```python
from build123d import *

# Parameters (mm, degrees)
BOSS_EXTRUDE1_DEPTH  = 7.1
SKETCH2_R            = 0.714611453
SKETCH2_R_2          = 0.75
BOSS_EXTRUDE2_DEPTH  = 0.48
SKETCH8_R            = 0.75
BOSS_EXTRUDE4_DEPTH  = 0.48
SKETCH9_R            = 0.75
BOSS_EXTRUDE5_DEPTH  = 0.48
SKETCH10_R           = 0.714611453
SKETCH10_R_2         = 0.75
BOSS_EXTRUDE7_DEPTH  = 0.48
SKETCH11_R           = 0.714611453
SKETCH11_R_2         = 0.75
BOSS_EXTRUDE8_DEPTH  = 0.48
SKETCH12_R           = 0.714611453
BOSS_EXTRUDE9_DEPTH  = 0.48
SKETCH13_R           = 0.75
BOSS_EXTRUDE10_DEPTH = 0.48
SKETCH15_R           = 1.5875
CUT_EXTRUDE3_DEPTH   = 8.1


with BuildPart() as part:
    # Sketch1 → Boss-Extrude1 (new body)
    with BuildSketch(Plane.XY):
        Polygon((-0.007801135, 4.977998784), (-3.525492932, 3.514460461), (-4.977998784, -0.007801135), (-3.514460461, -3.525492932), (0.007801135, -4.977998784), (3.525492932, -3.514460461), (4.977998784, 0.007801135), (3.514460461, 3.525492932), align=None)
    extrude(amount=BOSS_EXTRUDE1_DEPTH)

    # Sketch2 → Boss-Extrude2 (add)
    with BuildSketch(Plane(origin=(1.753329663, 4.251745858, 0), x_dir=(0.924478109, -0.381235132, 0), z_dir=(0.381235132, 0.924478109, 0))):
        with Locations((0, -1.25)):
            Circle(SKETCH2_R)
        with Locations((0, -3.55)):
            Circle(SKETCH2_R_2)
        with Locations((0, -5.85)):
            Circle(SKETCH2_R_2)
    extrude(amount=BOSS_EXTRUDE2_DEPTH)

    # Sketch8 → Boss-Extrude4 (add)
    with BuildSketch(Plane(origin=(4.246229622, 1.766647033, 0), x_dir=(0, 0, -1), z_dir=(0.923278687, 0.384130793, 0))):
        with Locations((-3.55, 0)):
            Circle(SKETCH8_R)
        with Locations((-5.85, 0)):
            Circle(SKETCH8_R)
    extrude(amount=BOSS_EXTRUDE4_DEPTH)

    # Sketch9 → Boss-Extrude5 (add)
    with BuildSketch(Plane(origin=(4.251745858, -1.753329663, 0), x_dir=(0, 0, -1), z_dir=(0.924478109, -0.381235132, 0))):
        with Locations((-5.85, 0)):
            Circle(SKETCH9_R)
    extrude(amount=BOSS_EXTRUDE5_DEPTH)

    # Sketch10 → Boss-Extrude7 (add)
    with BuildSketch(Plane(origin=(1.766647033, -4.246229622, 0), x_dir=(0.923278687, 0.384130793, 0), z_dir=(0.384130793, -0.923278687, 0))):
        with Locations((0, 5.85)):
            Circle(SKETCH10_R)
        with Locations((0, 1.25)):
            Circle(SKETCH10_R_2)
    extrude(amount=BOSS_EXTRUDE7_DEPTH)

    # Sketch11 → Boss-Extrude8 (add)
    with BuildSketch(Plane(origin=(-1.766647033, 4.246229622, 0), x_dir=(0.923278687, 0.384130793, 0), z_dir=(-0.384130793, 0.923278687, 0))):
        with Locations((-0.048036035, -1.25)):
            Circle(SKETCH11_R)
        with Locations((-0.048036035, -3.55)):
            Circle(SKETCH11_R_2)
    extrude(amount=BOSS_EXTRUDE8_DEPTH)

    # Sketch12 → Boss-Extrude9 (add)
    with BuildSketch(Plane(origin=(-4.251745858, 1.753329663, 0), x_dir=(0, 0, 1), z_dir=(-0.924478109, 0.381235132, 0))):
        with Locations((1.25, 0)):
            Circle(SKETCH12_R)
    extrude(amount=BOSS_EXTRUDE9_DEPTH)

    # Sketch13 → Boss-Extrude10 (add)
    with BuildSketch(Plane(origin=(-1.753329663, -4.251745858, 0), x_dir=(0.924478109, -0.381235132, 0), z_dir=(-0.381235132, -0.924478109, 0))):
        with Locations((0, 3.55)):
            Circle(SKETCH13_R)
    extrude(amount=BOSS_EXTRUDE10_DEPTH)

    # Sketch15 → Cut-Extrude3 (cut, through all)
    with BuildSketch(Plane.XY.offset(7.1)):
        Circle(SKETCH15_R)
    extrude(amount=-CUT_EXTRUDE3_DEPTH, mode=Mode.SUBTRACT)


solid = part.part
```
Geometry check sheet. Reference: the model listing, model coordinates, mm. Round coordinates to 2 decimals unless told otherwise and drop trailing zeros. Loops run counter-clockwise (first coordinate to the right, second up) from the corner with the lowest first, then second, coordinate; pieces in that order, holes last. Notation, with made-up numbers: (46, -33.75) - (95, -33.75) arc R19 ccw to (95, -23.75) - close; hole circle Ø4 at (54, 24.5). An arc over 180 degrees is marked (long way). Write item = value, one per line. Start each with the question number.
1. Section check A-A on x = -0.25. Enter the section's corners in (y, z).
2. Section check C-C on y = 3.75. Enter the section's corners in (x, z).
3. Section check B-B on z = 6. Enter the section's corners in (x, y) (1 decimal), then the cut area to 3 significant figures.
4. Section check D-D on z = 0.75. Enter the section's corners in (x, y) (1 decimal).
5. Thickness scan on line 1 (Y direction, x = 0, z = 3.5); line 2 (Y direction, x = 0.75, z = 1.5); line 3 (X direction, y = 0.5, z = 4.75). Record the ranges inside material, lowest first.
6. Depth check by flat-ended pin: pin 1 (3 mm diameter, centred on x = -2.5, z = 4.5, fed in from +Y); pin 2 (1.5 mm diameter, centred on y = 1, z = 3.5, fed in from -X); pin 3 (3 mm diameter, centred on y = -0.5, z = 6, fed in from +X). Enter the tip coordinate at first touch or a pass-through.
7. Mould release check, pull along Z, two halves, no side actions. Record for faces 1 (the face through (1.941, -4.693, 1.26)), 2 (the face through (-1.182, -4.743, 3.775)), 3 (the face through (1.742, -4.256, 3.5)): released by +Z, released by -Z, zero draft, split by the parting line, or undercut.
Working result:
q1.outline = (-4.87, 0) - (-1.57, 0) - (-1.57, 7.1) - (-4.87, 7.1) - close; (1.57, 0) - (4.88, 0) - (4.88, 7.1) - (1.57, 7.1) - close
q2.outline = (-2.96, 0) - (2.97, 0) - (2.97, 7.1) - (-2.96, 7.1) - close
q3.outline = (-5, 0) - (-3.5, -3.5) - (0, -5) - (1.1, -4.5) - (1.3, -5) - (2.6, -4.4) - (2.4, -4) - (3.5, -3.5) - (4, -2.4) - (4.4, -2.6) - (5, -1.3) - (4.5, -1.1) - (5, 0) - (4.5, 1.1) - (5, 1.3) - (4.4, 2.6) - (4, 2.4) - (3.5, 3.5) - (2.4, 4) - (2.6, 4.4) - (1.3, 5) - (1.1, 4.5) - (0, 5) - (-3.5, 3.5) - close; hole circle Ø3.2 at (0, 0)
q3.area = 65.0 mm^2
q4.outline = (-5, 0) - (-3.5, -3.5) - (0, -5) - (1.3, -4.5) - (1.4, -4.9) - (2.5, -4.5) - (2.3, -4) - (3.5, -3.5) - (5, 0) - (3.5, 3.5) - (2.2, 4.1) - (2.4, 4.5) - (1.5, 4.9) - (1.3, 4.4) - (0, 5) - (-1.3, 4.4) - (-1.5, 4.9) - (-2.5, 4.5) - (-2.3, 4) - (-3.5, 3.5) - (-4.1, 2.2) - (-4.5, 2.4) - (-4.9, 1.5) - (-4.4, 1.3) - close; hole circle Ø3.2 at (0, 0)
q5.line_1 = -4.97 to -1.59, 1.59 to 4.97
q5.line_2 = -4.67 to -1.4, 1.4 to 4.67
q5.line_3 = -4.77 to -1.51, 1.51 to 4.77
q6.pin_1 = 4.96
q6.pin_2 = -4.87
q6.pin_3 = 4.98
q7.face_1 = zero draft
q7.face_2 = split by the parting line
q7.face_3 = undercut
